The drawing under review shows one solid part. Ordinate dimensions are in mm from its lowest x, y, z. A direction names the side the tool comes from. Give positions to 0.01 mm unless a question says otherwise; leave off trailing zeros. Write each loop counter-clockwise with the first axis right and the second up, starting at its lowest first coordinate (ties: lowest second). Pieces come first, ordered by that corner, then holes. Notation, with made-up numbers: (56, -24.75) -> (101, -24.75) arc R20 cw to (101, -18.75) -> close; hole circle Ø3 at (47, -39.5). An arc over 180 degrees is marked (long way). Write item = value, one per line.
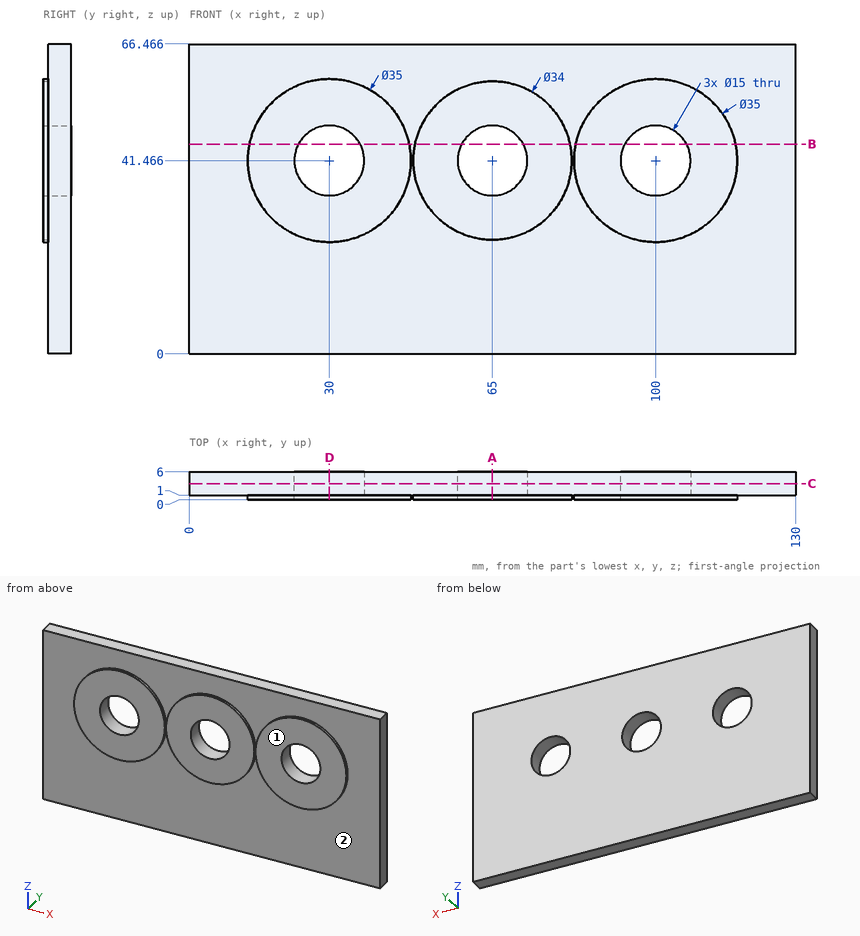
(1) Take a section at B-B (z = 45). Write out the cut boundary in (x, y) (1 decimal).
Answers below:
outline = (0, 1) -> (12.9, 1) -> (12.9, 0) -> (23.4, 0) -> (23.4, 6) -> (0, 6) -> close; (36.6, 0) -> (47.1, 0) -> (47.1, 1) -> (48.4, 1) -> (48.4, 0) -> (58.4, 0) -> (58.4, 6) -> (36.6, 6) -> close; (71.6, 0) -> (81.6, 0) -> (81.6, 1) -> (82.9, 1) -> (82.9, 0) -> (93.4, 0) -> (93.4, 6) -> (71.6, 6) -> close; (106.6, 0) -> (117.1, 0) -> (117.1, 1) -> (130, 1) -> (130, 6) -> (106.6, 6) -> close
(2) Take a section at A-A (x = 65). Write out the cut boundary in (y, z), plus the area to 3 significant figures.
Answers below:
outline = (0, 24.47) -> (1, 24.47) -> (1, 0) -> (6, 0) -> (6, 33.97) -> (0, 33.97) -> close; (0, 48.97) -> (6, 48.97) -> (6, 66.47) -> (1, 66.47) -> (1, 58.47) -> (0, 58.47) -> close
area = 276 mm^2
(3) To check wall thickness, follow probe 1 along X at (y, z) = (0.9, 57) (1 decimal); probe 2 along Z at (x, y) = (100, 2); probe 3 along Y at (x, z) = (11, 61). State the ranges of each line that lie inside material, in increasing order.
Answers below:
probe_1 = 21.9 to 38.1, 58.1 to 71.9, 91.9 to 108.1
probe_2 = 0 to 33.97, 48.97 to 66.47
probe_3 = 1 to 6
(4) Tool access review of the marked faces 1 and 2: name each direction out of +Z, -Z, +X, -X, +Y, -Y from which nothing blocks a thin tool from reaching the whole face with its end or side.
Answers below:
face_1 = +Z, -Z, +X, -X, -Y
face_2 = -Y
(5) Take a section at D-D (x = 30). Write out the cut boundary in (y, z).
Answers below:
outline = (0, 23.97) -> (1, 23.97) -> (1, 0) -> (6, 0) -> (6, 33.97) -> (0, 33.97) -> close; (0, 48.97) -> (6, 48.97) -> (6, 66.47) -> (1, 66.47) -> (1, 58.97) -> (0, 58.97) -> close
(6) Take a section at C-C (y = 3.45). Write out the cut boundary in (x, z).
Answers below:
outline = (0, 0) -> (130, 0) -> (130, 66.47) -> (0, 66.47) -> close; hole circle Ø15 at (30, 41.47); hole circle Ø15 at (65, 41.47); hole circle Ø15 at (100, 41.47)
